CAD build for the part. Positions are in the model's coordinates, mm. A direction names the side the tool comes from. Give positions to 0.01 mm unless a question says otherwise; leave off trailing zeros. Order: outer loops, then holes, each group sorted by start corner. A loop starts at its lowest first (then second) coordinate and runs counter-clockwise, first axis right, second up. Notation, with made-up numbers: M 57,76 L 61,76 A4 cw 61,80 Z; hole C 88.25,55 d11. An arc over 180 degrees is marked long. Put each result on its own line as item: value. Start each with the question number.
1) Pin check, flat tips, straight feed: pin 1 (5 mm diameter, centred on y = 15, z = 26, fed in from +X); pin 2 (2 mm diameter, centred on x = 114.5, y = 11.5, fed in from -Z); pin 3 (1.1 mm diameter, centred on x = 115.5, z = 25, fed in from +Y). Stop position of each tip, or through.
2) Cut at D-D (y = 50). Write the cut outline in (x, z), and give its area (3 significant figures).
3) Cut at A-A (z = 13). Give the number of separate pieces and of enclosed holes in the cut face, and give its area (3 significant figures).
4) Tool access for faces 1 (the face through (115, 53, 6)), 2 (the face through (114.8, 80, 19)), 3 (the face through (115, 35.1, 27.2)): list every direction of +Z, -Z, +X, -X, +Y, -Y with a clear straight run to the whole face (end or side of a thin tool).
5) Two-plate mould, pull along Z, no slides. Class faces 4 (the face through (115, 42, 33.8)), 5 (the face through (114.972, 41.536, 13.325)), 6 (the face through (115, 21, 4)): released by +Z, released by -Z, zero draft, split by the parting line, or undercut.
6) Cut at B-B (y = 64). Write the cut outline in (x, z).
7) Drill centre lines: line 1 (Z direction, x = 116.15, y = 57); line 2 (Y direction, x = 116.4, z = 6.5); line 3 (Z direction, x = 113.95, y = 36). Where is each one in solid material? Low to high. Write a range as [from, to].
```python
from build123d import *

# Parameters (mm, degrees)
CYLINDER007_R     = 1.5
CYLINDER007_DEPTH = 10
ARRAY014_Y_COUNT  = 8
ARRAY014_Y_PITCH  = 7
BOX052_W          = 10
BOX052_H          = 14
BOX052_DEPTH      = 13
BOX053_W          = 10
BOX053_H          = 30
BOX053_DEPTH      = 4
CYLINDER006_R     = 1.5
CYLINDER006_DEPTH = 10
ARRAY013_Y_COUNT  = 5
ARRAY013_Y_PITCH  = 7
BOX051_W          = 10
BOX051_H          = 10
BOX051_DEPTH      = 50
BOX050_W          = 10
BOX050_H          = 10
BOX050_DEPTH      = 50
BOX049_W          = 10
BOX049_H          = 10
BOX049_DEPTH      = 50
BOX048_W          = 10
BOX048_H          = 10
BOX048_DEPTH      = 50
BOX046_W          = 2
BOX046_H          = 80
BOX046_DEPTH      = 29.8
BOX047_W          = 4
BOX047_H          = 76
BOX047_DEPTH      = 29.8


with BuildPart() as array014:
    # Cylinder007 → Cylinder007 (new body)
    with BuildSketch(Plane(origin=(110, 25, 13), x_dir=(0, 0, -1), z_dir=(1, 0, 0))):
        Circle(CYLINDER007_R)
    extrude(amount=CYLINDER007_DEPTH)

    # Array014 Y: Array014 ×8


with BuildPart() as array014_1:
    add(array014.part)
    with Locations(*[(0, i * ARRAY014_Y_PITCH, 0) for i in range(1, ARRAY014_Y_COUNT)]):
        add(array014.part)


with BuildPart() as array014_2:
    # Array014 placement: moved
    add(array014_1.part.moved(Location((0, -10, 13))))


with BuildPart() as cube012:
    # Box052 → Box052 (new body)
    with BuildSketch(Plane(origin=(111, 5, 4), x_dir=(1, 0, 0), z_dir=(0, 0, 1))):
        with Locations((5, 7)):
            Rectangle(BOX052_W, BOX052_H)
    extrude(amount=BOX052_DEPTH)


with BuildPart() as cube013:
    # Box053 → Box053 (new body)
    with BuildSketch(Plane(origin=(111, 23, 4), x_dir=(1, 0, 0), z_dir=(0, 0, 1))):
        with Locations((5, 15)):
            Rectangle(BOX053_W, BOX053_H)
    extrude(amount=BOX053_DEPTH)


with BuildPart() as fusion008032:
    # Cylinder006 → Cylinder006 (new body)
    with BuildSketch(Plane(origin=(110, 25, 13), x_dir=(0, 0, -1), z_dir=(1, 0, 0))):
        Circle(CYLINDER006_R)
    extrude(amount=CYLINDER006_DEPTH)

    # Array013 Y: Fusion008032 ×5


with BuildPart() as fusion008032_1:
    add(fusion008032.part)
    with Locations(*[(0, i * ARRAY013_Y_PITCH, 0) for i in range(1, ARRAY013_Y_COUNT)]):
        add(fusion008032.part)


with BuildPart() as fusion008032_2:
    # Array013 placement: moved
    add(fusion008032_1.part.moved(Location((0, 4, 0))))

    # Fusion008032: union Array014, Cube012, Cube013
    add(array014_2.part)
    add(cube012.part)
    add(cube013.part)


with BuildPart() as obj1:
    # Box051 → Box051 (new body)
    with BuildSketch(Plane(origin=(110, 80.8, 0), x_dir=(1, 0, 0), z_dir=(0, 0, 1))):
        with Locations((5, 5)):
            Rectangle(BOX051_W, BOX051_H)
    extrude(amount=BOX051_DEPTH)


with BuildPart() as obj2:
    # Box050 → Box050 (new body)
    with BuildSketch(Plane(origin=(109, -8.8, 0), x_dir=(1, 0, 0), z_dir=(0, 0, 1))):
        with Locations((5, 5)):
            Rectangle(BOX050_W, BOX050_H)
    extrude(amount=BOX050_DEPTH)


with BuildPart() as obj3:
    # Box049 → Box049 (new body)
    with BuildSketch(Plane(origin=(114.8, 78.8, 0), x_dir=(1, 0, 0), z_dir=(0, 0, 1))):
        with Locations((5, 5)):
            Rectangle(BOX049_W, BOX049_H)
    extrude(amount=BOX049_DEPTH)


with BuildPart() as obj4:
    # Box048 → Box048 (new body)
    with BuildSketch(Plane(origin=(114.8, -6.8, 0), x_dir=(1, 0, 0), z_dir=(0, 0, 1))):
        with Locations((5, 5)):
            Rectangle(BOX048_W, BOX048_H)
    extrude(amount=BOX048_DEPTH)


with BuildPart() as obj5:
    # Box046 → Box046 (new body)
    with BuildSketch(Plane(origin=(113, 1, 23), x_dir=(1, 0, 0), z_dir=(0, 0, 1))):
        with Locations((1, 40)):
            Rectangle(BOX046_W, BOX046_H)
    extrude(amount=BOX046_DEPTH)


with BuildPart() as frontcover:
    # Box047 → Box047 (new body)
    with BuildSketch(Plane(origin=(113, 3, 23), x_dir=(1, 0, 0), z_dir=(0, 0, 1))):
        with Locations((2, 38)):
            Rectangle(BOX047_W, BOX047_H)
    extrude(amount=BOX047_DEPTH)

    # Fusion008031: union obj5
    add(obj5.part)


with BuildPart() as frontcover_1:
    # Fusion008031 placement: moved
    add(frontcover.part.moved(Location((0, 0, -19))))

    # Cut047: cut obj4
    add(obj4.part, mode=Mode.SUBTRACT)

    # Cut048: cut obj3
    add(obj3.part, mode=Mode.SUBTRACT)

    # Cut049: cut obj2
    add(obj2.part, mode=Mode.SUBTRACT)

    # Cut050: cut obj1
    add(obj1.part, mode=Mode.SUBTRACT)

    # Cut051: cut Fusion008032
    add(fusion008032_2.part, mode=Mode.SUBTRACT)


solid = frontcover_1.part
```
Solution:
1. pin 1: x = 117
1. pin 2: z = 17
1. pin 3: y = 78.8
2. outline: M 113,8 L 117,8 L 117,11.5 L 113,11.5 Z; M 113,14.5 L 117,14.5 L 117,24.5 L 113,24.5 Z; M 113,27.5 L 117,27.5 L 117,33.8 L 113,33.8 Z
2. area: 79.2 mm²
3. separate pieces: 7
3. enclosed holes: 0
3. area: 194 mm²
4. face 1: -Z, +X, -X
4. face 2: +Z, -Z, +X, +Y
4. face 3: +X, -X
5. face 4: released by +Z
5. face 5: undercut
5. face 6: released by -Z
6. outline: M 113,4 L 117,4 L 117,24.5 L 113,24.5 Z; M 113,27.5 L 117,27.5 L 117,33.8 L 113,33.8 Z
7. line 1: [4, 11.5], [14.5, 24.5], [27.5, 33.8]
7. line 2: [3.2, 5], [19, 23], [53, 78.8]
7. line 3: [8, 11.5], [14.5, 24.5], [27.5, 33.8]
